Design review of the part built by this model. Coordinates are the model's own, in mm. Face numbers are marked on the shaded views. A direction names the side the tool comes from. Round coordinates to 2 decimals unless told otherwise and drop trailing zeros. Order: outer loops, then holes, each group sorted by start corner. A loop starts at its lowest first (then second) coordinate and runs counter-clockwise, first axis right, second up. Notation, with made-up numbers: M 76.25,62 L 106.25,62 A8 ccw 106.25,76 Z; hole C 81.5,-18.75 d7. An arc over 180 degrees is marked long. Write each question's results on one line, items separated by ' | '. Start each with the question number.
Item 1: The part is to be moulded in two halves that separate along Y. For the marked faces 1, 2 and 3, say which applies: +Y half, -Y half, draft (parallel to the pull), parting line (faces both ways), or undercut.
Item 2: Take a section at C-C, the plane y = 86.5. Write out the cut boundary in (x, z).
Item 3: Take a section at B-B, the plane x = 66.5. Write out the cut boundary in (y, z).
Item 4: Wall thickness on line 1 (Y direction, x = 11, z = 5); line 2 (X direction, y = 17, z = 7.5); line 3 (Y direction, x = 47.5, z = 3): over which ranges is each line inside the solid? List them lowest first. Write a range as [from, to].
Item 5: Take a section at A-A, the plane z = 14. Write out the cut boundary in (x, y) (3 decimals), plus the area to 3 significant figures.
Item 6: Clearance check with flat-ended pins moving along their axes: pin 1 (10 mm diameter, centred on x = 32.5, z = 4, fed in from +Y); pin 2 (20.5 mm diameter, centred on x = -61.5, y = 16, fed in from +Z) (3 decimals); pin 3 (8 mm diameter, centred on y = -3, z = 8.5, fed in from -X). State where each tip first meets the part, or that it passes through.
Item 7: Machinability: for the marked faces 4 and 5, which of the approach directions +Z, -Z, +X, -X, +Y, -Y give a long, thin tool a straight path to every point of the face, cutting with its end or side? Answer none if there is none.
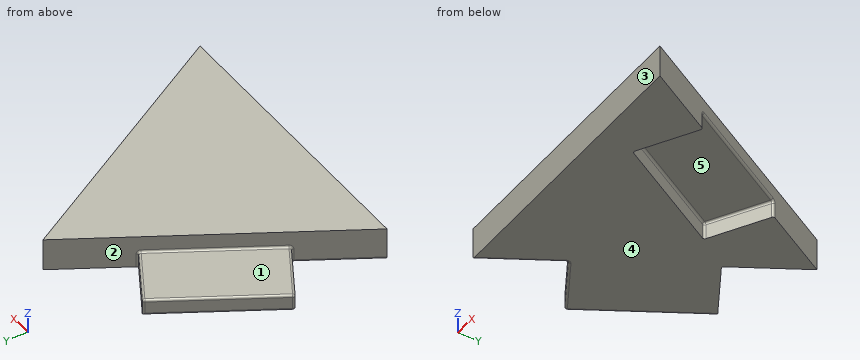
```python
from build123d import *

# Parameters (mm, degrees)
F1_DEPTH = 19.2024
F2_W     = 77.47
F2_H     = 10.16
F3_DEPTH = 39.37
F4_F1_R  = 1.27
F4_F2_R  = 1.27
F5_W     = 76.2
F5_H     = 9.525
F6_DEPTH = 38.1
F7_R     = 1.27


with BuildPart() as f1:
    # F0 (on Top) → F1 (new body)
    with BuildSketch(Plane.XY):
        Polygon((-85.725, -49.4933518263), (85.725, -49.4933518263), (0, 98.9867036526), align=None)
    extrude(amount=F1_DEPTH)

    # F2 (on face) → F3 (cut)
    with BuildSketch(Plane(origin=(42.8625, 24.7466759131, 0), x_dir=(-0.5, 0.8660254038, 0), z_dir=(0.8660254038, 0.5, 0))):
        with Locations((0, 5.08)):
            Rectangle(F2_W, F2_H)
    extrude(amount=-F3_DEPTH, mode=Mode.SUBTRACT)

    # F4: fillet of radius 1.27 on 6 edges, made by hand

    # F4_f1
    f4_f1_edges = [f1.edges().sort_by_distance(p)[0] for p in [
        (45.1822899265, -18.6413181024, 10.16),
        (28.134579853, -28.4838181024, 5.08),
        (8.767079853, 5.0616759131, 10.16),
        (6.4472899265, 48.4496699287, 10.16),
        (-10.600420147, 38.6071699287, 5.08),
    ]]
    fillet(f4_f1_edges, radius=F4_F1_R)

    # F4_f2
    f4_f2_edges = [f1.edges().sort_by_distance(p)[0] for p in [
        (62.23, -8.7988181024, 4.445),
        (62.0440128061, -8.476678833, 9.7880256121),
    ]]
    fillet(f4_f2_edges, radius=F4_F2_R)

    # F5 (on face) → F6 (join)
    with BuildSketch(Plane(origin=(-42.8625, 24.7466759131, 0), x_dir=(-0.5, -0.8660254038, 0), z_dir=(-0.8660254038, 0.5, 0))):
        with Locations((0, 4.7625)):
            Rectangle(F5_W, F5_H)
    extrude(amount=F6_DEPTH)

    # F7
    f7_edges = [f1.edges().sort_by_distance(p)[0] for p in [
        (-75.858068, 43.796676, 9.525),
        (-56.808068, 76.792244, 4.7625),
        (-75.858068, 43.796676, 0),
        (-94.908068, 10.801108, 4.7625),
        (-40.310284, 67.267244, 9.525),
        (-78.410284, 1.276108, 0),
        (-23.8125, 57.742244, 4.7625),
        (-61.9125, -8.248892, 4.7625),
        (-78.410284, 1.276108, 9.525),
        (-73.81875, -28.871122, 0),
        (-42.8625, 24.746676, 9.525),
    ]]
    fillet(f7_edges, radius=F7_R)


solid = f1.part
```
Results list:
1) face 1: draft | face 2: undercut | face 3: -Y half
2) outline: M -7.21,0 L 7.21,0 L 7.21,19.2 L -7.21,19.2 Z
3) outline: M -49.49,0 L -16.19,0 L -16.19,19.2 L -49.49,19.2 Z
4) line 1: [-49.49, 1.19], [51.08, 79.93] | line 2: [-91.33, 1.87] | line 3: [-49.49, -17.3]
5) outline: M -85.725,-49.493 L 85.725,-49.493 L 0,98.987 Z | area: 12,700 mm²
6) pin 1: y = -23.08 | pin 2: z = 9.525 | pin 3: x = -77.92
7) face 4: -Z, +X, -X, +Y, -Y | face 5: -Z
